from build123d import *

# Parameters (mm, degrees)
F0_W           = 40
F0_H           = 40
F1_DEPTH       = 10
F3_DEPTH       = 8.5
F4_W           = 16
F4_H           = 16
F5_DEPTH       = 2.5
F7_D           = 4.4
F7_CBORE_D     = 8.25
F7_CBORE_DEPTH = 2
F8_W           = 6
F8_H           = 10
F8_W_2         = 10
F8_H_2         = 6
F9_DEPTH       = 6
F11_D          = 3.2
F12_W          = 3
F12_H          = 6
F12_W_2        = 6
F12_H_2        = 3
F13_DEPTH      = 8
F15_D          = 3.2
F16_R          = 30
F17_R          = 8


with BuildPart() as f1:
    # F0 (on Top) → F1 (new body)
    with BuildSketch(Plane.XY):
        with Locations((20, 20)):
            Rectangle(F0_W, F0_H)
    extrude(amount=F1_DEPTH)

    # F2 (on face) → F3 (cut)
    with BuildSketch(Plane.XY.offset(10)):
        Polygon((40, 4), (40, 40), (4, 40), (4, 16), (11, 16), (16, 11), (16, 4), align=None)
    extrude(amount=-F3_DEPTH, mode=Mode.SUBTRACT)

    # F4 (on face) → F5 (cut)
    with BuildSketch(Plane.XY.offset(10)):
        with Locations((8, 8)):
            Rectangle(F4_W, F4_H)
    extrude(amount=-F5_DEPTH, mode=Mode.SUBTRACT)

    # F7 (through all)
    with Locations(Plane(origin=(0, 0, 0), x_dir=(1, 0, 0), z_dir=(0, 0, -1))):
        with Locations((9, -9)):
            CounterBoreHole(F7_D / 2, F7_CBORE_D / 2, F7_CBORE_DEPTH)

    # F8 (on face) → F9 (join)
    with BuildSketch(Plane.XY.offset(10)):
        with Locations((3, 35)):
            Rectangle(F8_W, F8_H)
        with Locations((35, 3)):
            Rectangle(F8_W_2, F8_H_2)
    extrude(amount=F9_DEPTH)

    # F11 (through all)
    with Locations(Plane(origin=(0, 0, 0), x_dir=(0, -1, 0), z_dir=(-1, 0, 0))):
        with Locations((-35, 11.5)):
            Hole(F11_D / 2)

    # F12 (on face) → F13 (cut)
    with BuildSketch(Plane.XY.offset(16)):
        with Locations((3, 35)):
            Rectangle(F12_W, F12_H)
        with Locations((35, 3)):
            Rectangle(F12_W_2, F12_H_2)
    extrude(amount=-F13_DEPTH, mode=Mode.SUBTRACT)

    # F15 (through all)
    with Locations(Plane.XZ):
        with Locations((35, 11.5)):
            Hole(F15_D / 2)

    # F16
    f16_edges = [f1.edges().sort_by_distance(p)[0] for p in [
        (40, 40, 0.75),
    ]]
    fillet(f16_edges, radius=F16_R)

    # F17
    f17_edges = [f1.edges().sort_by_distance(p)[0] for p in [
        (0, 0, 3.75),
    ]]
    fillet(f17_edges, radius=F17_R)


solid = f1.part
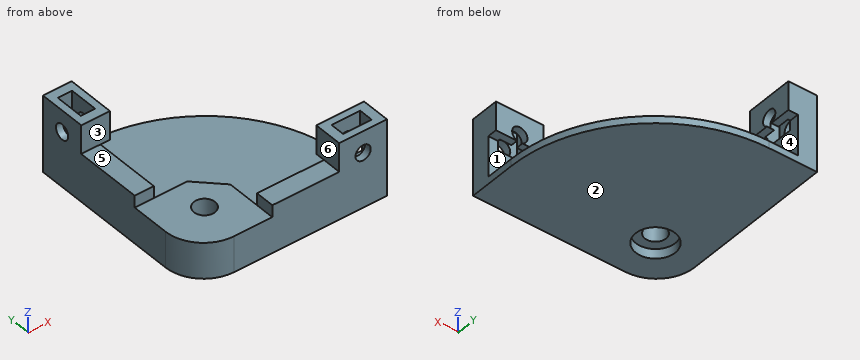
For this review, take the finished solid that the model builds, in its own axes (mm). Face numbers are marked on the shaded views. A direction names the side the tool comes from. Coordinates: 2 decimals unless noted, no trailing zeros. Loops run counter-clockwise (first coordinate to the right, second up) from the corner with the lowest first, then second, coordinate; pieces in that order, holes last. Notation, with made-up numbers: (-1, -25.5) - (30, -25.5) arc R19 cw to (30, 4.5) - close; hole circle Ø11 at (-5.5, 78.25). An arc over 180 degrees is marked (long way). Use a Markdown table: item, result. Add a question column.
Item 1: Tool access review of the marked faces 4, 5 and 6: name each direction out of +Z, -Z, +X, -X, +Y, -Y from which nothing blocks a thin tool from reaching the whole face with its end or side.
Item 2: Insertion check: pin 1 Ø17.5 at (x, y) = (11, 6.5) entering from +Z; pin 2 Ø1.8 at (y, z) = (6.5, 5) entering from +X; pin 3 Ø3 at (x, z) = (8, 5) entering from +Y; pin 4 Ø3 at (y, z) = (35, 11.5) entering from +X. Each pin has a flat end and moves straight along its axis. Give the tip position at first contact, or say it passes through.
Item 3: We need section C-C (z = 6.75). Give the boundary of the cut face in (x, y).
Item 4: We need section B-B (y = 9). Give the boundary of the cut face in (x, z) (3 decimals).
Item 5: We need section D-D (x = 35). Give the boundary of the cut face in (y, z).
Item 6: Mouldability with a two-part tool opening along Z and no side actions: class the marked faces 1, 2 and 3 as pulls with the +Z half, pulls with the -Z half, needs draft (parallel to the pull), parting line crosses it, or undercut.
Item 7: We need section A-A (z = 14.5). Give the boundary of the cut face in (x, y).
Item 8: For line 1 (Y direction, x = 5.35, z = 11.5); line 2 (X direction, y = 37.5, z = 12.5); line 3 (Z direction, x = 35, y = 5), list the stretches that pass through material, from the lowest coordinate up.
Results list:
| question | item | result |
|---|---|---|
| 1 | face 4 | +X, +Y |
| 1 | face 5 | +Z, +X, -X, -Y |
| 1 | face 6 | +Z, -X, +Y, -Y |
| 2 | pin 1 | stops at z = 10 |
| 2 | pin 2 | stops at x = 16 |
| 2 | pin 3 | stops at y = 16 |
| 2 | pin 4 | passes through |
| 3 | outline | (0, 8) arc R8 ccw to (8, 0) - (40, 0) - (40, 4) - (16, 4) - (16, 11) - (11, 16) - (4, 16) - (4, 40) - (0, 40) - close; hole circle Ø4.4 at (9, 9) |
| 4 | outline | (0, 0) - (4.875, 0) - (4.875, 2) - (6.8, 2) - (6.8, 7.5) - (0, 7.5) - close; (11.2, 2) - (13.125, 2) - (13.125, 0) - (40, 0) - (40, 1.5) - (16, 1.5) - (16, 7.5) - (11.2, 7.5) - close |
| 5 | outline | (0, 0) - (26.58, 0) - (26.58, 1.5) - (4, 1.5) - (4, 8) - (1.5, 8) - (1.5, 9.9) - (0, 9.9) - close; (0, 13.1) - (1.5, 13.1) - (1.5, 16) - (0, 16) - close; (4.5, 13.1) - (6, 13.1) - (6, 16) - (4.5, 16) - close |
| 6 | face 1 | undercut |
| 6 | face 2 | pulls with the -Z half |
| 6 | face 3 | needs draft |
| 7 | outline | (0, 30) - (6, 30) - (6, 40) - (0, 40) - close; (30, 0) - (40, 0) - (40, 6) - (30, 6) - close; hole (1.5, 32) - (4.5, 32) - (4.5, 38) - (1.5, 38) - close; hole (32, 1.5) - (38, 1.5) - (38, 4.5) - (32, 4.5) - close |
| 8 | line 1 | y = 30 to 33.4, 36.6 to 40 |
| 8 | line 2 | x = 0 to 1.5, 4.5 to 6 |
| 8 | line 3 | z = 0 to 1.5, 13.1 to 16 |
